Verification items for the finished model (mm, model axes). Face numbers are marked on the shaded views. Round coordinates to 2 decimals unless told otherwise and drop trailing zeros. Order: outer loops, then holes, each group sorted by start corner. A loop starts at its lowest first (then second) coordinate and runs counter-clockwise, first axis right, second up. Notation, with made-up numbers: M 21.5,-14 L 42.5,-14 A22 cw 42.5,8 Z; hole C 55.25,73 d10. An arc over 180 degrees is marked long. Use one line per item in the form item = value. Start each with the question number.
Item 1: Cross-section at A-A on y = 10. Enter the section's corners in (x, z).
Item 2: Cross-section at C-C on z = 6.5. Enter the section's corners in (x, y), then the cut area to 3 significant figures.
Item 3: Cross-section at D-D on z = 26. Enter the section's corners in (x, y).
Item 4: Go/stop test with flat-tipped pins: pin 1 Ø4 at (x, y) = (-7, 8.5) entering from -Z; pin 2 Ø6.5 at (x, y) = (-10, 10) entering from -Z; pin 3 Ø10 at (y, z) = (3, -11) entering from +X. Record where each tip stops, or that it passes through.
Item 5: Thickness scan on probe 1 along Y at (x, z) = (10, 24.5); probe 2 along X at (y, z) = (4.75, 7); probe 3 along Z at (x, y) = (-5.5, 1.5). Record the ranges inside material, lowest first. Write a range as [from, to].
Item 6: Release check for a two-part mould opening along Z. For the marked faces 1, 2 and 3 record: +Z half, -Z half, draft (parallel to the pull), parting line (faces both ways), or undercut.
Item 7: Cross-section at B-B on x = 0. Enter the section's corners in (y, z).
from build123d import *

# Parameters (mm, degrees)
SKETCH1_R           = 21.5
SKETCH1_R_2         = 18.25
BOSS_EXTRUDE1_DEPTH = 20
SKETCH2_R           = 2
CUT_EXTRUDE1_DEPTH  = 10


with BuildPart() as part:
    # Sketch1 → Boss-Extrude1 (new body)
    # profile 1 of 2: a face of its own
    with BuildSketch(Plane(origin=(0, 0, 0), x_dir=(1, 0, 0), z_dir=(0, 1, 0))):
        with BuildLine():
            ThreePointArc((21.5, 0), (0, -21.5), (-21.5, 0))
            Line((-21.5, 0), (-21.5, -30))
            Line((-21.5, -30), (21.5, -30))
            Line((21.5, -30), (21.5, 0))
        make_face()
    # profile 2 of 2: a face of its own
    with BuildSketch(Plane(origin=(0, 0, 0), x_dir=(1, 0, 0), z_dir=(0, 1, 0))):
        Circle(SKETCH1_R)
        with Locations(Location((0, 0, 0), (0, 0, 270))):
            Circle(SKETCH1_R_2, mode=Mode.SUBTRACT)
    extrude(amount=BOSS_EXTRUDE1_DEPTH)

    # Sketch2 → Cut-Extrude1 (cut)
    with BuildSketch(Plane.XY.offset(30)):
        with Locations((-10, 10)):
            Circle(SKETCH2_R)
        with Locations((10, 10)):
            Circle(SKETCH2_R)
    extrude(amount=-CUT_EXTRUDE1_DEPTH, mode=Mode.SUBTRACT)


solid = part.part
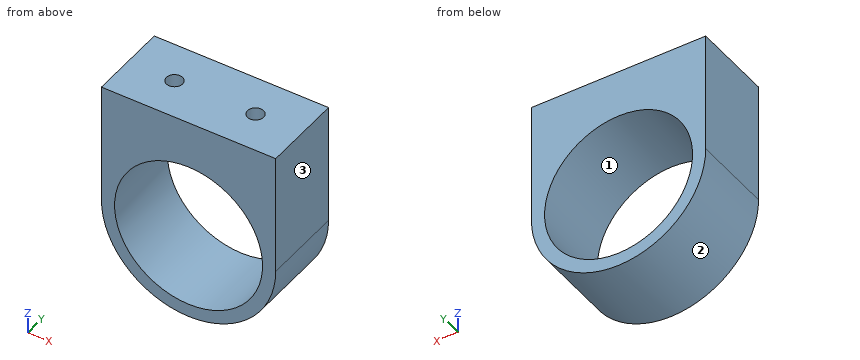
Output values:
q1.outline = M -21.5,0 A21.5 ccw 21.5,0 L 21.5,30 L 12,30 L 12,20 L 8,20 L 8,30 L -8,30 L -8,20 L -12,20 L -12,30 L -21.5,30 Z; hole C 0,0 d36.5
q2.outline = M -21.5,0 L -17.05,0 L -17.05,20 L -21.5,20 Z; M 17.05,0 L 21.5,0 L 21.5,20 L 17.05,20 Z
q2.area = 178 mm2
q3.outline = M -21.5,0 L 21.5,0 L 21.5,20 L -21.5,20 Z; hole C -10,10 d4; hole C 10,10 d4
q4.pin_1 = -20.91
q4.pin_2 = -20.41
q4.pin_3 = 20.65
q5.probe_1 = [0, 8], [12, 20]
q5.probe_2 = [-21.5, -16.85], [16.85, 21.5]
q5.probe_3 = [-20.78, -17.4], [17.4, 30]
q6.face_1 = undercut
q6.face_2 = -Z half
q6.face_3 = draft
q7.outline = M 0,-21.5 L 20,-21.5 L 20,-18.25 L 0,-18.25 Z; M 0,18.25 L 20,18.25 L 20,30 L 0,30 Z
